Could you check a few things on this drawing? It's one solid part, dimensions in mm from its lowest x, y, z. Round coordinates to 2 decimals unless told otherwise and drop trailing zeros. Write each loop counter-clockwise with the first axis right and the second up, starting at its lowest first coordinate (ties: lowest second). Pieces come first, ordered by that corner, then holes. Notation, with made-up numbers: (53.25, 43.5) -> (93.25, 43.5) arc R8 ccw to (93.25, 53.5) -> close; hole circle Ø8 at (-9, 28.5). An arc over 180 degrees is marked (long way). Answer in a Markdown table with one row per item.
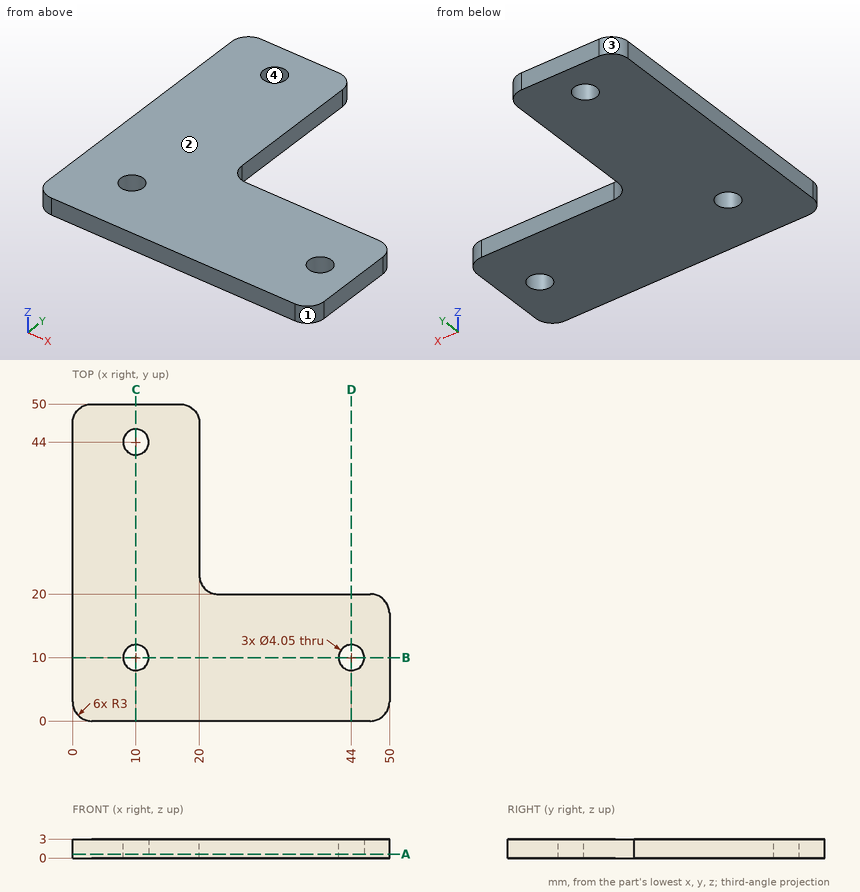
1) Imagine slicing it at D-D, the plane x = 44. Please give me the cut outline in (y, z) (3 decimals).
Findings:
| item | result |
|---|---|
| outline | (0, 0) -> (7.975, 0) -> (7.975, 3) -> (0, 3) -> close; (12.025, 0) -> (20, 0) -> (20, 3) -> (12.025, 3) -> close |
2) Please list where these lines run through material, in increasing order: line 1 (Y direction, x = 10, z = 2.05) (3 decimals); line 2 (Y direction, x = 44, z = 1.15) (3 decimals); line 3 (Y direction, x = 11, z = 0.7).
Findings:
| item | result |
|---|---|
| line 1 | y = 0 to 7.975, 12.025 to 41.975, 46.025 to 50 |
| line 2 | y = 0 to 7.975, 12.025 to 20 |
| line 3 | y = 0 to 8.24, 11.76 to 42.24, 45.76 to 50 |
3) Thinking about a two-plate mould opening in Y: for the marked faces 1, 2, 3 and 4, which applies, +Y half, -Y half, draft (parallel to the pull), parting line (faces both ways), or undercut?
Findings:
| item | result |
|---|---|
| face 1 | -Y half |
| face 2 | draft |
| face 3 | +Y half |
| face 4 | undercut |
4) Imagine slicing it at B-B, the plane y = 10. Please give me the cut outline in (x, z) (3 decimals).
Findings:
| item | result |
|---|---|
| outline | (0, 0) -> (7.975, 0) -> (7.975, 3) -> (0, 3) -> close; (12.025, 0) -> (41.975, 0) -> (41.975, 3) -> (12.025, 3) -> close; (46.025, 0) -> (50, 0) -> (50, 3) -> (46.025, 3) -> close |
5) Imagine slicing it at A-A, the plane z = 0.6. Please give me the cut outline in (x, y) (3 decimals), plus the area to 3 significant figures.
Findings:
| item | result |
|---|---|
| outline | (0, 3) arc R3 ccw to (3, 0) -> (47, 0) arc R3 ccw to (50, 3) -> (50, 17) arc R3 ccw to (47, 20) -> (23, 20) arc R3 cw to (20, 23) -> (20, 47) arc R3 ccw to (17, 50) -> (3, 50) arc R3 ccw to (0, 47) -> close; hole circle Ø4.05 at (10, 10); hole circle Ø4.05 at (10, 44); hole circle Ø4.05 at (44, 10) |
| area | 1,550 mm^2 |
6) For pin 1 (0.9 mm diameter, centred on y = 31, z = 2, fed in from +X); pin 2 (4 mm diameter, centred on x = 19, y = 30, fed in from -Z); pin 3 (2.5 mm diameter, centred on x = 10, y = 10, fed in from -Z); pin 4 (1.5 mm diameter, centred on x = 40, z = 2, fed in from +Y), each with a flat end and sliding along its axis, tell me the tip position at first contact or that it passes through.
Findings:
| item | result |
|---|---|
| pin 1 | stops at x = 20 |
| pin 2 | stops at z = 0 |
| pin 3 | passes through |
| pin 4 | stops at y = 20 |
